The figure shows three views and two pictorial views of one solid part (mm, origin at its lowest corner). Answer the questions. A direction names the side the tool comes from. Round coordinates to 2 decimals unless told otherwise and drop trailing zeros. Write each loop counter-clockwise with the first axis right and the second up, starting at its lowest first coordinate (ties: lowest second). Pieces come first, ordered by that corner, then holes. Notation, with made-up numbers: M -21,-9.5 L 7,-9.5 A24 ccw 7,1.5 Z; hole C 54.25,-34 d7. An arc over 180 degrees is marked long. Answer in a Markdown table with one row per item.
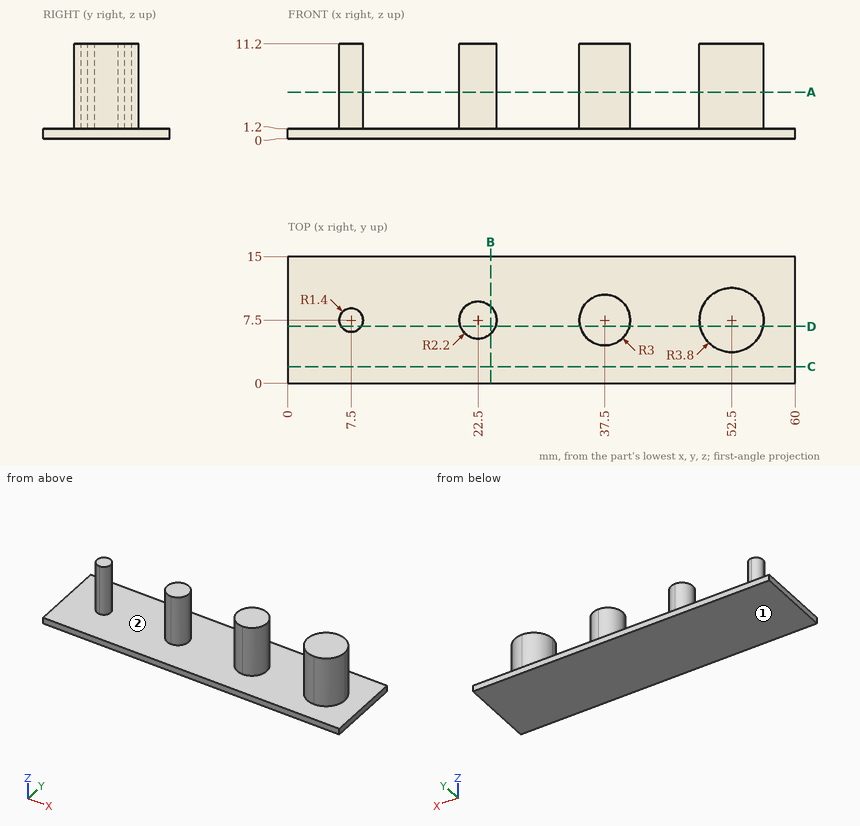
1. The part is cut by section A-A (z = 5.5). Determine the outline of the cut face in (x, y), plus the area to 3 significant figures.
Calculated:
| item | result |
|---|---|
| outline | C 7.5,7.5 d2.8; C 22.5,7.5 d4.4; C 37.5,7.5 d6; C 52.5,7.5 d7.6 |
| area | 95.0 mm² |
2. Consider line 1 along X through (y, z) = (8.5, 10); line 2 along X through (y, z) = (9, 10); line 3 along X through (y, z) = (5.5, 7.25). Determine where each line is inside the solid, lowest interval first. Write a range as from..to.
Calculated:
| item | result |
|---|---|
| line 1 | x = 6.52..8.48, 20.54..24.46, 34.67..40.33, 48.83..56.17 |
| line 2 | x = 20.89..24.11, 34.9..40.1, 49.01..55.99 |
| line 3 | x = 21.58..23.42, 35.26..39.74, 49.27..55.73 |
3. The part is cut by section B-B (x = 24). Determine the outline of the cut face in (y, z).
Calculated:
| item | result |
|---|---|
| outline | M 0,0 L 15,0 L 15,1.2 L 9.11,1.2 L 9.11,11.2 L 5.89,11.2 L 5.89,1.2 L 0,1.2 Z |
4. The part is cut by section C-C (y = 2). Determine the outline of the cut face in (x, z).
Calculated:
| item | result |
|---|---|
| outline | M 0,0 L 60,0 L 60,1.2 L 0,1.2 Z |
5. A tool of negligible diameter and unlimited length cuts with its end or side. For the marked faces 1 and 2, from which of +Z, -Z, +X, -X, +Y, -Y can it reach the whole face along a straight path? Write none if from no direction.
Calculated:
| item | result |
|---|---|
| face 1 | -Z, +X, -X, +Y, -Y |
| face 2 | +Z |
6. Given pin 1 (1 mm diameter, centred on x = 43.5, y = 3, fed in from -Z); pin 2 (3 mm diameter, centred on x = 17, z = 4, fed in from +Y); pin 3 (1.5 mm diameter, centred on y = 10, z = 9, fed in from -X); pin 4 (1.5 mm diameter, centred on x = 40.5, z = 2, fed in from +Y), each flat-ended and moving along its own axis, determine where each tip first touches the part or whether it passes through.
Calculated:
| item | result |
|---|---|
| pin 1 | stops at z = 0 |
| pin 2 | passes through |
| pin 3 | stops at x = 21.17 |
| pin 4 | stops at y = 9.48 |
7. The part is cut by section D-D (y = 6.75). Determine the outline of the cut face in (x, z).
Calculated:
| item | result |
|---|---|
| outline | M 0,0 L 60,0 L 60,1.2 L 56.23,1.2 L 56.23,11.2 L 48.77,11.2 L 48.77,1.2 L 40.4,1.2 L 40.4,11.2 L 34.6,11.2 L 34.6,1.2 L 24.57,1.2 L 24.57,11.2 L 20.43,11.2 L 20.43,1.2 L 8.68,1.2 L 8.68,11.2 L 6.32,11.2 L 6.32,1.2 L 0,1.2 Z |
